```python
from build123d import *

# Parameters (mm, degrees)
BOSS_EXTRUDE1_DEPTH   = 5
BOSS_EXTRUDE2_START   = -15
BOSS_EXTRUDE2_DEPTH   = 15
F_1_0MM_DOWEL_HOLE1_D = 4.5
SKETCH5_R             = 2.25
CUT_EXTRUDE1_DEPTH    = 81.039052968


with BuildPart() as part:
    # Sketch1 → Boss-Extrude1 (new body)
    with BuildSketch(Plane.XY):
        with BuildLine():
            Line((22.5, 25), (22.5, 5))
            Line((22.5, 5), (30, 5))
            Line((30, 5), (30, 12.5))
            Line((30, 12.5), (40, 12.5))
            ThreePointArc((40, 12.5), (48.838834765, 16.161165235), (52.5, 25))
            Line((52.5, 25), (47.5, 25))
            ThreePointArc((47.5, 25), (40, 17.5), (32.5, 25))
            Line((32.5, 25), (22.5, 25))
        make_face()
        with BuildLine():
            Line((15, 12.5), (15, 5))
            Line((15, 5), (22.5, 5))
            Line((22.5, 5), (22.5, 25))
            Line((22.5, 25), (12.5, 25))
            ThreePointArc((12.5, 25), (5, 17.5), (-2.5, 25))
            Line((-2.5, 25), (-7.5, 25))
            ThreePointArc((-7.5, 25), (-3.838834765, 16.161165235), (5, 12.5))
            Line((5, 12.5), (15, 12.5))
        make_face()
    extrude(amount=BOSS_EXTRUDE1_DEPTH)

    # Sketch1<3> → Boss-Extrude2 (add)
    with BuildSketch(Plane.XY.offset(BOSS_EXTRUDE2_START)):
        with BuildLine():
            Line((30, 12.5), (30, 5))
            Line((30, 5), (50, 5))
            Line((50, 5), (45, 0))
            Line((45, 0), (67.5, 0))
            Line((67.5, 0), (67.5, 15))
            Line((67.5, 15), (57.5, 15))
            Line((57.5, 15), (57.5, 25))
            Line((57.5, 25), (52.5, 25))
            ThreePointArc((52.5, 25), (48.838834765, 16.161165235), (40, 12.5))
            Line((40, 12.5), (30, 12.5))
        make_face()
        with BuildLine():
            Line((-22.5, 0), (0, 0))
            Line((0, 0), (-5, 5))
            Line((-5, 5), (15, 5))
            Line((15, 5), (15, 12.5))
            Line((15, 12.5), (5, 12.5))
            ThreePointArc((5, 12.5), (-3.838834765, 16.161165235), (-7.5, 25))
            Line((-7.5, 25), (-12.5, 25))
            Line((-12.5, 25), (-12.5, 15))
            Line((-12.5, 15), (-22.5, 15))
            Line((-22.5, 15), (-22.5, 0))
        make_face()
        with BuildLine():
            Line((15, 12.5), (15, 5))
            Line((15, 5), (22.5, 5))
            Line((22.5, 5), (22.5, 25))
            Line((22.5, 25), (12.5, 25))
            ThreePointArc((12.5, 25), (5, 17.5), (-2.5, 25))
            Line((-2.5, 25), (-7.5, 25))
            ThreePointArc((-7.5, 25), (-3.838834765, 16.161165235), (5, 12.5))
            Line((5, 12.5), (15, 12.5))
        make_face()
        with BuildLine():
            Line((22.5, 25), (22.5, 5))
            Line((22.5, 5), (30, 5))
            Line((30, 5), (30, 12.5))
            Line((30, 12.5), (40, 12.5))
            ThreePointArc((40, 12.5), (48.838834765, 16.161165235), (52.5, 25))
            Line((52.5, 25), (47.5, 25))
            ThreePointArc((47.5, 25), (40, 17.5), (32.5, 25))
            Line((32.5, 25), (22.5, 25))
        make_face()
    extrude(amount=BOSS_EXTRUDE2_DEPTH)

    # Mirror1: part across plane


with BuildPart() as part_1:
    add(part.part)
    add(part.part.mirror(Plane(origin=(0, 0, -15), x_dir=(1, 0, 0), z_dir=(0, 0, -1))))

    # Ø1.0mm Dowel Hole1 (through all)
    with Locations(Plane(origin=(-7.5, 25, -7.5), x_dir=(1, 0, 0), z_dir=(0, 1, 0))):
        with Locations((0, 0), (60, 15), (60, 0), (0, 15)):
            Hole(F_1_0MM_DOWEL_HOLE1_D / 2)

    # Sketch5 → Cut-Extrude1 (cut, through all)
    with BuildSketch(Plane(origin=(0, 25, 0), x_dir=(1, 0, 0), z_dir=(0, 1, 0))):
        with Locations(Location((22.5, 30, 0), (0, 0, 180))):
            Circle(SKETCH5_R)
        with Locations(Location((22.5, 0, 0), (0, 0, 180))):
            Circle(SKETCH5_R)
    extrude(amount=-CUT_EXTRUDE1_DEPTH, mode=Mode.SUBTRACT)


solid = part_1.part
```
Input: part model. Units: mm. Frame: model coordinates. A direction names the side the tool comes from. Give positions to 0.01 mm unless a question says otherwise; leave off trailing zeros. Loops run counter-clockwise (first coordinate to the right, second up) from the corner with the lowest first, then second, coordinate; pieces in that order, holes last. Notation, with made-up numbers: (16, 83.25) -> (63, 83.25) arc R35 ccw to (63, 118.25) -> close; hole circle Ø6 at (-21.5, 85.5). An arc over 180 degrees is marked (long way). Use a Markdown table: item, result.
Q1. Ray query, probe 1 along Z at (x, y) = (22.5, 16.5); probe 2 along Z at (x, y) = (52.5, 17.5); probe 3 along X at (y, z) = (21, -4). Return the intervals inside material, ascending. Write a range as from..to.
Entries:
| item | result |
|---|---|
| probe 1 | z = -35..-32.25, -27.75..-2.25, 2.25..5 |
| probe 2 | z = -30..-24.75, -20.25..-9.75, -5.25..0 |
| probe 3 | x = -12.5..-1.34, 11.34..33.66, 46.34..57.5 |
Q2. First-contact query: P1, Ø2.5, axis at y = 8.5, z = 2, coming from the +X side; P2, Ø6, axis at x = 55.5, y = 4.5, coming from the -Z side; P3, Ø1.5, axis at x = 33, z = -32, coming from the -Y side; P4, Ø4, axis at x = 52.5, z = -22.5, coming from the -Y side. Flat tips, straight axial feed; report the tip coordinate or a pass-through.
Entries:
| item | result |
|---|---|
| P1 | stops at x = 30 |
| P2 | stops at z = -30 |
| P3 | stops at y = 12.5 |
| P4 | passes through |
Q3. Pull-direction query (Z, two-part tool) for faces 1 (the cylindrical face through (20.42, 15.14, -30.86)), 2 (the flat face through (22, 15, 5)), 3 (the flat face through (-22.5, 8, -15)); classes: pulls with the +Z half, pulls with the -Z half, needs draft (parallel to the pull), parting line crosses it, or undercut.
Entries:
| item | result |
|---|---|
| face 1 | undercut |
| face 2 | pulls with the +Z half |
| face 3 | needs draft |
Q4. Section query C-C, the plane y = 22.5. State how many separate pieces and enclosed holes the cut face has, plus the area to 3 significant figures.
Entries:
| item | result |
|---|---|
| separate pieces | 3 |
| enclosed holes | 6 |
| area | 1,470 mm² |
Q5. Access query for faces 4 (the flat face through (10, 12.5, -32)), 5 (the flat face through (30, 9, -32)), 6 (the flat face through (-17, 15, -15)). Directions: +Z, -Z, +X, -X, +Y, -Y. A direction counts if a zero-diameter tool reaches every point of the face in a straight line with its end or side. Return the directions, or none.
Entries:
| item | result |
|---|---|
| face 4 | -Z, -X, -Y |
| face 5 | -Z, +X, -Y |
| face 6 | +Z, -Z, -X, +Y |
Q6. Section query B-B, the plane y = 9. Return the cut outline in (x, z).
Entries:
| item | result |
|---|---|
| outline | (-22.5, -30) -> (15, -30) -> (15, -35) -> (30, -35) -> (30, -30) -> (67.5, -30) -> (67.5, 0) -> (30, 0) -> (30, 5) -> (15, 5) -> (15, 0) -> (-22.5, 0) -> close; hole circle Ø4.5 at (-7.5, -22.5); hole circle Ø4.5 at (-7.5, -7.5); hole circle Ø4.5 at (22.5, -30); hole circle Ø4.5 at (22.5, 0); hole circle Ø4.5 at (52.5, -22.5); hole circle Ø4.5 at (52.5, -7.5) |
Q7. Section query A-A, the plane x = 22.5. Return the cut outline in (y, z).
Entries:
| item | result |
|---|---|
| outline | (5, -35) -> (25, -35) -> (25, -32.25) -> (5, -32.25) -> close; (5, -27.75) -> (25, -27.75) -> (25, -2.25) -> (5, -2.25) -> close; (5, 2.25) -> (25, 2.25) -> (25, 5) -> (5, 5) -> close |
Q8. Section query D-D, the plane z = -1. Return the cut outline in (x, y), plus the area to 3 significant figures.
Entries:
| item | result |
|---|---|
| outline | (-22.5, 0) -> (0, 0) -> (-5, 5) -> (20.48, 5) -> (20.48, 25) -> (12.5, 25) arc R7.5 cw to (-2.5, 25) -> (-12.5, 25) -> (-12.5, 15) -> (-22.5, 15) -> close; (24.52, 5) -> (50, 5) -> (45, 0) -> (67.5, 0) -> (67.5, 15) -> (57.5, 15) -> (57.5, 25) -> (47.5, 25) arc R7.5 cw to (32.5, 25) -> (24.52, 25) -> close |
| area | 1,540 mm² |
